Geometry check sheet. Reference: the model listing, model coordinates, mm. A direction names the side the tool comes from. Give positions to 0.01 mm unless a question says otherwise; leave off trailing zeros. Write each loop counter-clockwise with the first axis right and the second up, starting at its lowest first coordinate (ties: lowest second). Pieces come first, ordered by that corner, then holes.
(1) Tool access check on faces 4 (the cylindrical face through (4.47, -5.06, 7.44)), 5 (the cylindrical face through (-6.7, 0.83, 7.44)), 6 (the cylindrical face through (7.5, -1.5, 7.4)), 7 (the cylindrical face through (0.58, -7.64, 7.44)). Record the directions out of +Z, -Z, +X, -X, +Y, -Y that give a thin tool (end or side, any length) a straight path to the whole face; none if there is none.
(2) Cross-section at B-B (y = 7.5). Record the boundary of the cut face in (x, z).
(3) Cross-section at D-D (x = -0.5). Record the boundary of the cut face in (y, z).
(4) Cross-section at A-A (x = -3.5). Record the boundary of the cut face in (y, z).
(5) Mould release check, pull along X, two halves, no side actions. Record for faces 1 (the cylindrical face through (-3, -7, 7)), 2 (the flat face through (0, 0, 0)), 3 (the cylindrical face through (6.619, -3.864, 7.437)): +X half, -X half, draft (parallel to the pull), parting line (faces both ways), or undercut.
(6) Cross-section at C-C (y = -7). Record the boundary of the cut face in (x, z).
(7) Thickness scan on line 1 along X through (y, z) = (4.5, 6.5); line 2 along Y through (x, z) = (-7, 10.5); line 3 along X through (y, z) = (7.5, 11.5). Record the ranges inside material, lowest first.
(8) Depth check by flat-ended pin: P1, Ø2, axis at x = -7.5, z = 8.5, coming from the +Y side; P2, Ø4, axis at y = 6, z = 3, coming from the +X side. Enter the tip coordinate at first touch or a pass-through.
```python
from build123d import *

# Parameters (mm, degrees)
SKETCH1_R           = 9.25
BOSS_EXTRUDE1_DEPTH = 3
BOSS_EXTRUDE2_DEPTH = 9


with BuildPart() as part:
    # Sketch1 → Boss-Extrude1 (new body)
    with BuildSketch(Plane.XY):
        Circle(SKETCH1_R)
    extrude(amount=BOSS_EXTRUDE1_DEPTH)

    # Sketch2 → Boss-Extrude2 (add)
    with BuildSketch(Plane.XY.offset(3)):
        with BuildLine():
            Line((2.218704647, 8.205324472), (1.849752862, 8.296289192))
            ThreePointArc((1.849752862, 8.296289192), (1.25913347, 7.547573069), (0.822693575, 6.699677252))
            ThreePointArc((0.822693575, 6.699677252), (0.000453114, 6.749999985), (-0.821794095, 6.699787643))
            ThreePointArc((-0.821794095, 6.699787643), (-1.258120151, 7.547742047), (-1.848639018, 8.296537457))
            Line((-1.848639018, 8.296537457), (-2.217603012, 8.205622273))
            ThreePointArc((-2.217603012, 8.205622273), (-2.39262478, 7.268192553), (-2.385036281, 6.31459436))
            ThreePointArc((-2.385036281, 6.31459436), (-3.136480191, 5.977038732), (-3.841209099, 5.550460581))
            ThreePointArc((-3.841209099, 5.550460581), (-4.621620694, 6.098516089), (-5.492481762, 6.487113696))
            Line((-5.492481762, 6.487113696), (-5.776932761, 6.235146179))
            ThreePointArc((-5.776932761, 6.235146179), (-5.496261527, 5.323756714), (-5.046383068, 4.482914))
            ThreePointArc((-5.046383068, 4.482914), (-5.554883684, 3.834809938), (-5.98064939, 3.12958989))
            ThreePointArc((-5.98064939, 3.12958989), (-6.926363634, 3.252193589), (-7.878063126, 3.191570364))
            Line((-7.878063126, 3.191570364), (-8.012836833, 2.836273238))
            ThreePointArc((-8.012836833, 2.836273238), (-7.340770995, 2.159712371), (-6.551664309, 1.624252067))
            ThreePointArc((-6.551664309, 1.624252067), (-6.700730268, 0.814072401), (-6.74999498, -0.008232129))
            ThreePointArc((-6.74999498, -0.008232129), (-7.644360136, -0.339167268), (-8.458875168, -0.835123275))
            Line((-8.458875168, -0.835123275), (-8.413096553, -1.212355721))
            ThreePointArc((-8.413096553, -1.212355721), (-7.503598294, -1.49909605), (-6.556038214, -1.60650644))
            ThreePointArc((-6.556038214, -1.60650644), (-6.3115203, -2.393159313), (-5.972998067, -3.144168267))
            ThreePointArc((-5.972998067, -3.144168267), (-6.611125856, -3.852828992), (-7.101860851, -4.670500236))
            Line((-7.101860851, -4.670500236), (-6.886017241, -4.983248595))
            ThreePointArc((-6.886017241, -4.983248595), (-5.947441652, -4.814479631), (-5.058502772, -4.469233682))
            ThreePointArc((-5.058502772, -4.469233682), (-4.476417094, -5.052147068), (-3.827659279, -5.559813346))
            ThreePointArc((-3.827659279, -5.559813346), (-4.063362315, -6.483854026), (-4.117895799, -7.435921879))
            Line((-4.117895799, -7.435921879), (-3.781434364, -7.612539271))
            ThreePointArc((-3.781434364, -7.612539271), (-3.028797802, -7.02692395), (-2.402125307, -6.308113348))
            ThreePointArc((-2.402125307, -6.308113348), (-1.615820678, -6.553748816), (-0.805449879, -6.70177219))
            ThreePointArc((-0.805449879, -6.70177219), (-0.584731436, -7.629506241), (-0.190570445, -8.497863432))
            Line((-0.190570445, -8.497863432), (0.189429554, -8.49788894))
            ThreePointArc((0.189429554, -8.49788894), (0.583707123, -7.629584676), (0.804550118, -6.701880267))
            ThreePointArc((0.804550118, -6.701880267), (1.614940783, -6.55396569), (2.401278382, -6.308435791))
            ThreePointArc((2.401278382, -6.308435791), (3.027854368, -7.027330521), (3.7804123, -7.613046883))
            Line((3.7804123, -7.613046883), (4.116897444, -7.436474665))
            ThreePointArc((4.116897444, -7.436474665), (4.062491781, -6.484399498), (3.826912806, -5.560327183))
            ThreePointArc((3.826912806, -5.560327183), (4.475738772, -5.052748009), (5.057902704, -4.469912777))
            ThreePointArc((5.057902704, -4.469912777), (5.946795225, -4.815278068), (6.885348147, -4.98417304))
            Line((6.885348147, -4.98417304), (7.101233744, -4.671453662))
            ThreePointArc((7.101233744, -4.671453662), (6.610608531, -3.853716541), (5.972575889, -3.14497015))
            ThreePointArc((5.972575889, -3.14497015), (6.311198947, -2.394006651), (6.555822471, -1.607386614))
            ThreePointArc((6.555822471, -1.607386614), (7.503396964, -1.50010344), (8.412933711, -1.21348522))
            Line((8.412933711, -1.21348522), (8.458762972, -0.836258923))
            ThreePointArc((8.458762972, -0.836258923), (7.644314532, -0.340193567), (6.749993814, -0.009138357))
            ThreePointArc((6.749993814, -0.009138357), (6.700839502, 0.813172779), (6.551882316, 1.623372451))
            ThreePointArc((6.551882316, 1.623372451), (7.341060883, 2.158726808), (8.013217548, 2.83519744))
            Line((8.013217548, 2.83519744), (7.878491542, 3.190512657))
            ThreePointArc((7.878491542, 3.190512657), (6.926800198, 3.251263653), (5.981069502, 3.128786923))
            ThreePointArc((5.981069502, 3.128786923), (5.555398481, 3.834064126), (5.046984881, 4.482236452))
            ThreePointArc((5.046984881, 4.482236452), (5.496976224, 5.32301876), (5.777769815, 6.234370535))
            Line((5.777769815, 6.234370535), (5.493352647, 6.486376238))
            ThreePointArc((5.493352647, 6.486376238), (4.622439416, 6.097895553), (3.841954247, 5.549944825))
            ThreePointArc((3.841954247, 5.549944825), (3.137282617, 5.976617587), (2.385884033, 6.314274098))
            ThreePointArc((2.385884033, 6.314274098), (2.393600558, 7.267871263), (2.218704647, 8.205324472))
        make_face()
    extrude(amount=BOSS_EXTRUDE2_DEPTH)


solid = part.part
```
Reply:
1. face 4: +Z
1. face 5: +Z, -X
1. face 6: +Z, +X
1. face 7: +Z, -Y
2. outline: (-5.41, 0) - (5.41, 0) - (5.41, 3) - (2.37, 3) - (2.37, 12) - (1.23, 12) - (1.23, 3) - (-1.23, 3) - (-1.23, 12) - (-2.37, 12) - (-2.37, 3) - (-5.41, 3) - close
3. outline: (-9.24, 0) - (9.24, 0) - (9.24, 3) - (6.73, 3) - (6.73, 12) - (-7.86, 12) - (-7.86, 3) - (-9.24, 3) - close
4. outline: (-8.56, 0) - (8.56, 0) - (8.56, 3) - (5.77, 3) - (5.77, 12) - (-7.42, 12) - (-7.42, 3) - (-8.56, 3) - close
5. face 1: undercut
5. face 2: draft
5. face 3: +X half
6. outline: (-6.05, 0) - (6.05, 0) - (6.05, 3) - (4.11, 3) - (4.11, 12) - (3, 12) - (3, 3) - (0.75, 3) - (0.75, 12) - (-0.75, 12) - (-0.75, 3) - (-3, 3) - (-3, 12) - (-4.12, 12) - (-4.12, 3) - (-6.05, 3) - close
7. line 1: x = -5.06 to 5.06
7. line 2: y = -4.82 to -4.47, -1.58 to -0.08, 1.9 to 3.25
7. line 3: x = -2.37 to -1.23, 1.23 to 2.37
8. P1: stops at y = 3.25
8. P2: stops at x = 8.34
